from build123d import *

# Parameters (mm, degrees)
SKETCH1_W           = 187.96
SKETCH1_H           = 127
BOSS_EXTRUDE1_DEPTH = 127
CUT_EXTRUDE1_DEPTH  = 25.4
SKETCH6_R           = 4.699
CUT_EXTRUDE2_DEPTH  = 12.7
SKETCH7_W           = 182.88
SKETCH7_H           = 121.92
CUT_EXTRUDE4_DEPTH  = 99.06
CUT_EXTRUDE5_DEPTH  = 25.4
CUT_EXTRUDE6_DEPTH  = 3.048


with BuildPart() as part:
    # Sketch1 → Boss-Extrude1 (new body)
    with BuildSketch(Plane.XY):
        with Locations((93.98, 63.5)):
            Rectangle(SKETCH1_W, SKETCH1_H)
    extrude(amount=BOSS_EXTRUDE1_DEPTH)

    # Sketch3 → Cut-Extrude1 (cut)
    with BuildSketch(Plane(origin=(0, 0, 0), x_dir=(-1, 0, 0), z_dir=(0, 0, -1))):
        Polygon((-170.18, 0), (-132.08, 0), (-140.929239756, 25.412400336), (-161.150123966, 25.412400336), align=None)
    extrude(amount=-CUT_EXTRUDE1_DEPTH, mode=Mode.SUBTRACT)

    # Sketch6 → Cut-Extrude2 (cut)
    with BuildSketch(Plane.XZ.offset(-25.412400336)):
        with Locations(Location((151.039681861, 7.391433819, 0), (0, 0, 270))):
            Circle(SKETCH6_R)
    extrude(amount=-CUT_EXTRUDE2_DEPTH, mode=Mode.SUBTRACT)

    # Sketch7 → Cut-Extrude4 (cut)
    with BuildSketch(Plane.XY.offset(127)):
        with Locations((93.98, 63.5)):
            Rectangle(SKETCH7_W, SKETCH7_H)
    extrude(amount=-CUT_EXTRUDE4_DEPTH, mode=Mode.SUBTRACT)

    # Sketch9 → Cut-Extrude5 (cut)
    with BuildSketch(Plane.XY.offset(27.94)):
        Polygon((162.943164317, 27.952400336), (171.973040351, 2.54), (185.42, 2.54), (185.42, 124.46), (2.54, 124.46), (2.54, 2.54), (130.274896212, 2.54), (139.124135968, 27.952400336), align=None)
    extrude(amount=-CUT_EXTRUDE5_DEPTH, mode=Mode.SUBTRACT)

    # Sketch10 → Cut-Extrude6 (cut)
    with BuildSketch(Plane.XZ):
        with BuildLine():
            Line((39.281842654, 36.576), (66.929, 36.576))
            ThreePointArc((66.929, 36.576), (83.82, 19.685), (66.929, 2.794))
            Line((66.929, 2.794), (39.281842654, 2.794))
            ThreePointArc((39.281842654, 2.794), (22.390842654, 19.685), (39.281842654, 36.576))
        make_face()
    extrude(amount=-CUT_EXTRUDE6_DEPTH, mode=Mode.SUBTRACT)


solid = part.part
Could you check a few things on this model? Use its own coordinates, in mm. A direction names the side the tool comes from. Give positions to 0.01 mm unless a question says otherwise; leave off trailing zeros. Order: outer loops, then holes, each group sorted by start corner. A loop starts at its lowest first (then second) coordinate and runs counter-clockwise, first axis right, second up. Notation, with made-up numbers: (2, 0.5) -> (32, 0.5) arc R30 ccw to (32, 28.5) -> close; hole circle Ø4 at (53.25, 82.5). An arc over 180 degrees is marked (long way). Return JSON: item names as keys, results as strings.
1. Imagine slicing it at B-B on z = 83. List the corners of the cut face in (x, y) for me.
Answer list:
{"outline": "(0, 0) -> (187.96, 0) -> (187.96, 127) -> (0, 127) -> close; hole (2.54, 2.54) -> (185.42, 2.54) -> (185.42, 124.46) -> (2.54, 124.46) -> close"}
2. Imagine slicing it at C-C on y = 80.5. List the corners of the cut face in (x, z) for me.
Answer list:
{"outline": "(0, 0) -> (187.96, 0) -> (187.96, 127) -> (185.42, 127) -> (185.42, 2.54) -> (2.54, 2.54) -> (2.54, 127) -> (0, 127) -> close"}
3. On a 3-axis mill with a long thin cutter (end or side, diameter ignored), from which of +Z, -Z, +X, -X, +Y, -Y can I reach the whole of each face in a straight line? I mean faces 3 (the flat face through (93, 124.46, 66)), 4 (the flat face through (151, 13, 25.4)), 5 (the flat face through (93, 127, 63)), 6 (the cylindrical face through (22.395, 1.252, 19.314)). Say none if no direction works.
Answer list:
{"face 3": "+Z", "face 4": "-Z, -Y", "face 5": "+Z, -Z, +X, -X, +Y", "face 6": "-Y"}
4. Imagine slicing it at A-A on x = 42. List the corners of the cut face in (y, z) for me, then the cut area to 3 significant figures.
Answer list:
{"outline": "(0, 0) -> (127, 0) -> (127, 127) -> (124.46, 127) -> (124.46, 2.54) -> (2.54, 2.54) -> (2.54, 2.79) -> (0, 2.79) -> close; (0, 36.58) -> (2.54, 36.58) -> (2.54, 127) -> (0, 127) -> close", "area": "869 mm2"}
5. I need wall thicknesses on line 1 (Y direction, x = 149.5, z = 22); line 2 (Y direction, x = 67.5, z = 67.5); line 3 (X direction, y = 9.5, z = 6). Which ranges of each line are inside material? Lowest first, please. Write a range as from..to.
Answer list:
{"line 1": "y = 25.41..27.95, 124.46..127", "line 2": "y = 0..2.54, 124.46..127", "line 3": "x = 0..2.54, 132.7..135.39, 166.8..169.5, 185.42..187.96"}
6. For pin 1 Ø1 at (x, y) = (48.5, 47) entering from -Z; pin 2 Ø6 at (x, z) = (151, 16.5) entering from -Y; pin 3 Ø12 at (x, y) = (156, 39) entering from +Z; pin 4 Ø5 at (x, y) = (157.5, 15.5) entering from +Z, each with a flat end and sliding along its axis, tell me the tip position at first contact or that it passes through.
Answer list:
{"pin 1": "stops at z = 0", "pin 2": "stops at y = 25.41", "pin 3": "stops at z = 2.54", "pin 4": "stops at z = 27.94"}
7. Thinking about a two-plate mould opening in X: for faces 1 (the flat face through (136.443, 12.528, 12.522)), 2 (the flat face through (94, 125, 127)), which applies, pulls with the +X half, pulls with the -X half, needs draft (parallel to the pull), parting line crosses it, or undercut?
Answer list:
{"face 1": "undercut", "face 2": "needs draft"}
8. Imagine slicing it at D-D on x = 125.5. List the corners of the cut face in (y, z) for me, then the cut area to 3 significant figures.
Answer list:
{"outline": "(0, 0) -> (127, 0) -> (127, 127) -> (124.46, 127) -> (124.46, 2.54) -> (2.54, 2.54) -> (2.54, 127) -> (0, 127) -> close", "area": "955 mm2"}
